Design review of the part built by this model. Coordinates are the model's own, in mm. Coordinates: 2 decimals unless noted, no trailing zeros. Write each loop counter-clockwise with the first axis right and the second up, starting at its lowest first coordinate (ties: lowest second). Pieces come first, ordered by that corner, then holes.
Q1. Take a section at C-C, the plane x = 33.82. Write out the cut boundary in (y, z) (3 decimals).
Q2. Take a section at D-D, the plane y = 2.15. Write out the cut boundary in (x, z) (3 decimals).
Q3. Take a section at A-A, the plane x = 43.82. Write out the cut boundary in (y, z) (3 decimals), plus the area to 3 significant figures.
Q4. Take a section at B-B, the plane z = -32. Write out the cut boundary in (x, y), plus the area to 3 significant figures.
Q5. For L1, parallel to X at y = 0.9, z = -34; L2, parallel to Z at x = 44.5, y = 1.25 (3 decimals); L3, parallel to Z at x = 11, y = 4.3 (3 decimals), list the stretches that pass through material, from the lowest coordinate up.
Q6. For pin 1 Ø2 at (x, z) = (14.465, -26.675) entering from -Y, flat-tipped, find the tip position at first contact; note if it passes through.
from build123d import *

# Parameters (mm, degrees)
SKETCH1_W           = 50.8
SKETCH1_H           = 66.675
BOSS_EXTRUDE1_DEPTH = 5
SKETCH2_R           = 2.075
SKETCH2_R_2         = 1.85
CUT_EXTRUDE1_DEPTH  = 6
CUT_EXTRUDE2_REACH  = 7
SKETCH3_R           = 2.2
CUT_EXTRUDE3_REACH  = 7


with BuildPart() as part:
    # Sketch1 → Boss-Extrude1 (new body)
    with BuildSketch(Plane(origin=(0, 0, 0), x_dir=(1, 0, 0), z_dir=(0, 1, 0))):
        with Locations((25.4, 33.3375)):
            Rectangle(SKETCH1_W, SKETCH1_H)
    extrude(amount=BOSS_EXTRUDE1_DEPTH)

    # Sketch2 → Cut-Extrude1 (cut, through all)
    with BuildSketch(Plane(origin=(0, 5, 0), x_dir=(1, 0, 0), z_dir=(0, 1, 0))):
        with Locations(Location((12.465, 57.075, 0), (0, 0, 270))):  # turned: the seam where the file's is
            Circle(SKETCH2_R)
        with Locations(Location((12.465, 7.075, 0), (0, 0, 270))):  # turned: the seam where the file's is
            Circle(SKETCH2_R)
        with Locations(Location((14.465, 26.675, 0), (0, 0, 270))):  # turned: the seam where the file's is
            Circle(SKETCH2_R_2)
    extrude(amount=-CUT_EXTRUDE1_DEPTH, mode=Mode.SUBTRACT)

    # Sketch3 → Cut-Extrude2 (cut, up to next)
    with BuildSketch(Plane(origin=(0, 5, 0), x_dir=(1, 0, 0), z_dir=(0, 1, 0)), mode=Mode.PRIVATE) as cut_extrude2_sk1:
        with Locations(Location((43.82, 41.925, 0), (0, 0, 270))):  # turned: the seam where the file's is
            Circle(SKETCH3_R)
    cut_extrude2_tool1 = extrude(cut_extrude2_sk1.sketch, amount=-CUT_EXTRUDE2_REACH, mode=Mode.PRIVATE) & part.part
    add(cut_extrude2_tool1.solids().sort_by_distance((43.82, 5, -41.925))[0], mode=Mode.SUBTRACT)
    # Sketch3 → Cut-Extrude2 (cut, up to next)
    with BuildSketch(Plane(origin=(0, 5, 0), x_dir=(1, 0, 0), z_dir=(0, 1, 0)), mode=Mode.PRIVATE) as cut_extrude2_sk2:
        with Locations(Location((43.82, 11.425, 0), (0, 0, 270))):  # turned: the seam where the file's is
            Circle(SKETCH3_R)
    cut_extrude2_tool2 = extrude(cut_extrude2_sk2.sketch, amount=-CUT_EXTRUDE2_REACH, mode=Mode.PRIVATE) & part.part
    add(cut_extrude2_tool2.solids().sort_by_distance((43.82, 5, -11.425))[0], mode=Mode.SUBTRACT)

    # Sketch4 → Cut-Extrude3 (cut, up to next)
    with BuildSketch(Plane(origin=(0, 5, 0), x_dir=(1, 0, 0), z_dir=(0, 1, 0)), mode=Mode.PRIVATE) as cut_extrude3_sk1:
        with BuildLine():
            Line((38.21, 46.675), (38.21, 16.675))
            ThreePointArc((38.21, 16.675), (33.82, 12.285), (29.43, 16.675))
            Line((29.43, 16.675), (29.43, 46.675))
            ThreePointArc((29.43, 46.675), (33.82, 51.065), (38.21, 46.675))
        make_face()
    cut_extrude3_tool1 = extrude(cut_extrude3_sk1.sketch, amount=-CUT_EXTRUDE3_REACH, mode=Mode.PRIVATE) & part.part
    add(cut_extrude3_tool1.solids().sort_by_distance((33.82, 5, -31.675))[0], mode=Mode.SUBTRACT)


solid = part.part
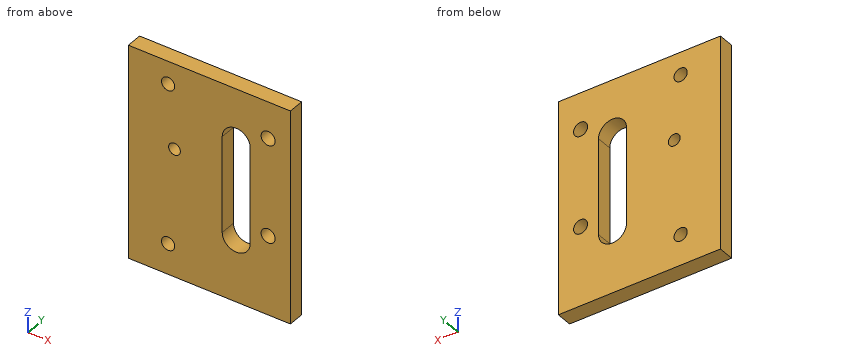
Responses:
1. outline: (0, -66.675) - (5, -66.675) - (5, -51.065) - (0, -51.065) - close; (0, -12.285) - (5, -12.285) - (5, 0) - (0, 0) - close
2. outline: (0, -66.675) - (50.8, -66.675) - (50.8, 0) - (0, 0) - close; hole circle Ø4.15 at (12.465, -57.075); hole circle Ø4.15 at (12.465, -7.075); hole circle Ø3.7 at (14.465, -26.675); hole (29.43, -46.675) arc R4.39 ccw to (38.21, -46.675) - (38.21, -16.675) arc R4.39 ccw to (29.43, -16.675) - close; hole circle Ø4.4 at (43.82, -41.925); hole circle Ø4.4 at (43.82, -11.425)
3. outline: (0, -66.675) - (5, -66.675) - (5, -44.125) - (0, -44.125) - close; (0, -39.725) - (5, -39.725) - (5, -13.625) - (0, -13.625) - close; (0, -9.225) - (5, -9.225) - (5, 0) - (0, 0) - close
3. area: 289 mm2
4. outline: (0, 0) - (29.43, 0) - (29.43, 5) - (0, 5) - close; (38.21, 0) - (50.8, 0) - (50.8, 5) - (38.21, 5) - close
4. area: 210 mm2
5. L1: x = 0 to 29.43, 38.21 to 50.8
5. L2: z = -66.675 to -44.017, -39.833 to -13.517, -9.333 to 0
5. L3: z = -66.675 to -58.544, -55.606 to -8.544, -5.606 to 0
6. pin 1: passes through
